The model under review builds one solid part; all positions refer to its coordinate system, in mm. A direction names the side the tool comes from. Give positions to 0.01 mm unless a question says otherwise; leave off trailing zeros. Write each loop counter-clockwise with the first axis right and the second up, starting at its lowest first coordinate (ties: lowest second). Pieces come first, ordered by that corner, then holes. Notation, with made-up numbers: (-0.75, 29) -> (50.25, 29) arc R24 ccw to (50.25, 64) -> close; hole circle Ø10 at (-19, 46). An arc over 180 degrees is marked (long way). Use CSV: the item, a comma, the result in double quotes.
```python
from build123d import *

# Parameters (mm, degrees)
SKETCH1_R           = 7.3025
BOSS_EXTRUDE1_DEPTH = 50.8
SKETCH2_R           = 1.6129
CUT_EXTRUDE1_DEPTH  = 50.8
SKETCH5_W           = 2.54
SKETCH5_H           = 3
SKETCH6_R           = 5.4229
CUT_EXTRUDE3_DEPTH  = 35.68192


with BuildPart() as part:
    # Sketch1 → Boss-Extrude1 (new body)
    with BuildSketch(Plane(origin=(0, 0, 0), x_dir=(1, 0, 0), z_dir=(0, 1, 0))):
        Circle(SKETCH1_R)
    extrude(amount=BOSS_EXTRUDE1_DEPTH)

    # Sketch2 → Cut-Extrude1 (cut)
    with BuildSketch(Plane(origin=(0, 50.8, 0), x_dir=(1, 0, 0), z_dir=(0, 1, 0))):
        Circle(SKETCH2_R)
    extrude(amount=-CUT_EXTRUDE1_DEPTH, mode=Mode.SUBTRACT)

    # Sketch3 → Cut-Revolve1 (revolve, cut)
    with BuildSketch(Plane.XY):
        Polygon((-5.4229, 15.118959148), (-1.6129, 9.215668113), (-1.6129, 15.118959148), align=None)
    revolve(axis=Axis((0, 34.671, 0), (0, -1, 0)), mode=Mode.SUBTRACT)

    # Sketch5 → Revolve1 (revolve)
    with BuildSketch(Plane(origin=(0, 0, 0), x_dir=(0, 0, -1), z_dir=(1, 0, 0))):
        with Locations((8.5725, 49.3)):
            Rectangle(SKETCH5_W, SKETCH5_H)
    revolve(axis=Axis((0, 34.671, 0), (0, -1, 0)))

    # Sketch6 → Cut-Extrude3 (cut)
    with BuildSketch(Plane(origin=(0, 50.8, 0), x_dir=(1, 0, 0), z_dir=(0, 1, 0))):
        Circle(SKETCH6_R)
    extrude(amount=-CUT_EXTRUDE3_DEPTH, mode=Mode.SUBTRACT)


solid = part.part
```
Q1. Machinability: for faces 1 (the cylindrical face through (6.746, 23.565, 2.797)), 2 (the cylindrical face through (1.54, 4.67, -0.48)), which of the approach directions +Z, -Z, +X, -X, +Y, -Y give a long, thin tool a straight path to every point of the face, cutting with its end or side? Answer none if there is none.
Derived:
face 1,"-Y"
face 2,"+Y, -Y"
Q2. Consider section D-D (z = -6.75). Write out the cut boundary in (x, y), then the cut area to 3 significant figures.
Derived:
outline,"(-7.16, 47.8) -> (-2.79, 47.8) -> (-2.79, 0) -> (2.79, 0) -> (2.79, 47.8) -> (7.16, 47.8) -> (7.16, 50.8) -> (-7.16, 50.8) -> close"
area,"309 mm2"
Q3. The part is to be moulded in two halves that separate along X. For faces 3 (the cylindrical face through (-1.176, 33.209, 5.294)), 4 (the flat face through (-4, 50.8, 4)), 5 (the cylindrical face through (-6, 49.3, 7.8)), say which applies: pulls with the +X half, pulls with the -X half, needs draft (parallel to the pull), parting line crosses it, or undercut.
Derived:
face 3,"undercut"
face 4,"needs draft"
face 5,"parting line crosses it"
Q4. Consider section C-C (y = 41). Write out the cut boundary in (x, z) (1 decimal), then the cut area to 3 significant figures.
Derived:
outline,"circle Ø14.6 at (0, 0); hole circle Ø10.8 at (0, 0)"
area,"75.1 mm2"
Q5. To check wall thickness, follow probe 1 along X at (y, z) = (6.75, 0); probe 2 along X at (y, z) = (30, 0). State the ranges of each line that lie inside material, in increasing order.
Derived:
probe 1,"x = -7.3 to -1.61, 1.61 to 7.3"
probe 2,"x = -7.3 to -5.42, 5.42 to 7.3"
Q6. Insertion check: pin 1 (4 mm diameter, centred on y = 41, z = -4, fed in from -X); pin 2 (3.5 mm diameter, centred on x = -2, z = -0.5, fed in from +Y); pin 3 (10 mm diameter, centred on x = 1.5, z = -3.5, fed in from -Y); pin 4 (2 mm diameter, centred on y = 20, z = 4.5, fed in from +X). Each pin has a flat end and moves straight along its axis. Give the tip position at first contact, or say it passes through.
Derived:
pin 1,"stops at x = -7.02"
pin 2,"stops at y = 12.62"
pin 3,"stops at y = 0"
pin 4,"stops at x = 6.41"
